Geometry check sheet. Reference: drawing and pictorial views, mm from the part's lowest x, y, z. Give positions to 0.01 mm unless a question says otherwise; leave off trailing zeros. Write each loop counter-clockwise with the first axis right and the second up, starting at its lowest first coordinate (ties: lowest second). Pieces come first, ordered by that corner, then holes. Notation, with made-up numbers: (10.25, -25.5) -> (48.25, -25.5) arc R7 ccw to (48.25, -14.5) -> close; hole circle Ø1 at (-9, 61). An arc over 180 degrees is marked (long way). Use a Markdown table: item, result. Add a question column.
1. Gauge pin test, flat ends, axial feed: P1, Ø1.5, axis at y = 3.5, z = 14, coming from the +X side; P2, Ø1, axis at x = 6, y = 3.5, coming from the +Z side; P3, Ø2, axis at y = 4.5, z = 10, coming from the +X side; P4, Ø3, axis at x = 7.94, z = 7.94, coming from the -Y side. Record the tip position at first contact, or that the pin passes through.
2. Cross-section at B-B (y = 3.85). Enter the section's corners in (x, z) (1 decimal).
3. Cross-section at A-A (y = 0.45). Enter the section's corners in (x, z).
4. Release check for a two-part mould opening along X. For the marked faces 1 and 2 record: released by +X, released by -X, zero draft, split by the parting line, or undercut.
5. Scan lines: probe 1 along Y at (x, z) = (4.25, 9.5) (1 decimal); probe 2 along X at (y, z) = (0.6, 7.25) (1 decimal); probe 3 along Z at (x, y) = (6.5, 1.45) (1 decimal). Record each from-to range of solid material in increasing order. Write a range as [from, to].
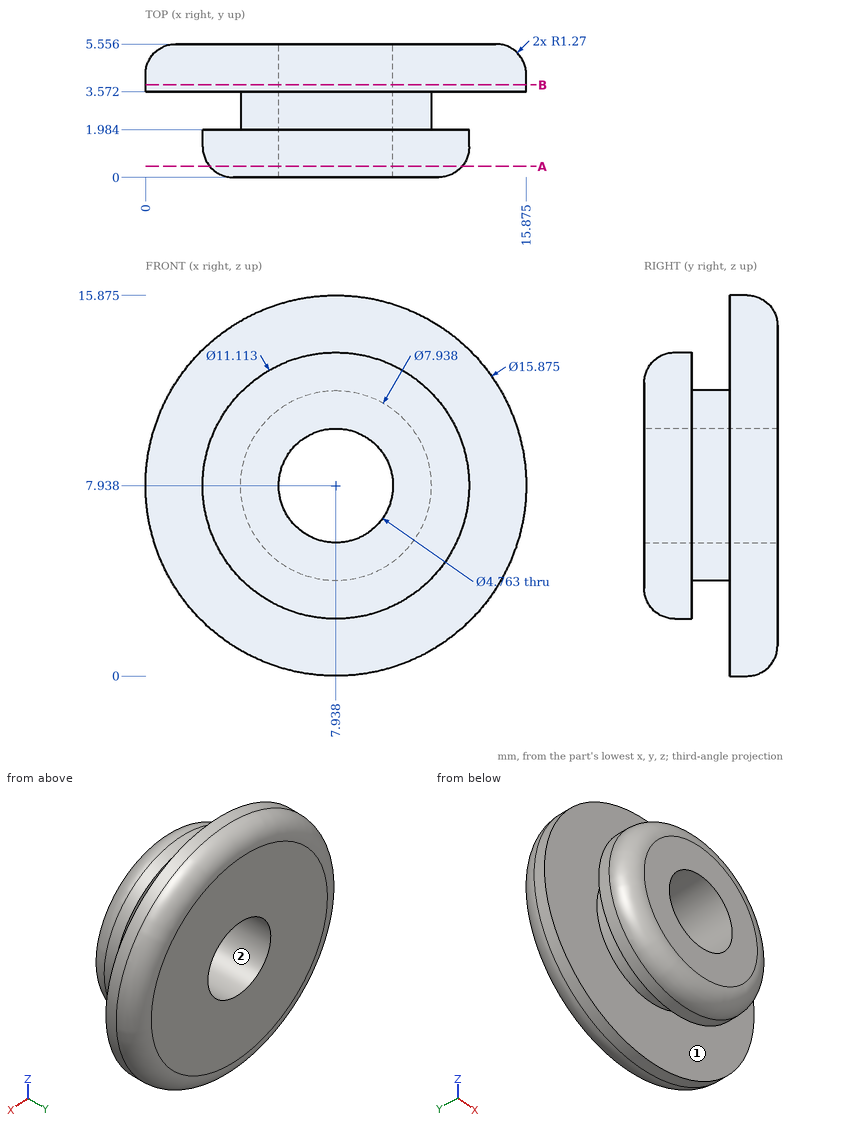
Worked answers:
| question | item | result |
|---|---|---|
| 1 | P1 | stops at x = 13.83 |
| 1 | P2 | stops at z = 15.74 |
| 1 | P3 | stops at x = 15.8 |
| 1 | P4 | passes through |
| 2 | outline | circle Ø15.9 at (7.9, 7.9); hole circle Ø4.8 at (7.9, 7.9) |
| 3 | outline | circle Ø10.51 at (7.94, 7.94); hole circle Ø4.76 at (7.94, 7.94) |
| 4 | face 1 | zero draft |
| 4 | face 2 | undercut |
| 5 | probe 1 | y = [0, 2], [3.6, 5.6] |
| 5 | probe 2 | x = [2.6, 5.7], [10.2, 13.3] |
| 5 | probe 3 | z = [2.6, 6], [9.8, 13.3] |
